Work out the finished part from the listing and answer in its coordinate system (mm). Give positions to 0.01 mm unless a question says otherwise; leave off trailing zeros. Order: outer loops, then holes, each group sorted by start corner. A loop starts at its lowest first (then second) coordinate and runs counter-clockwise, first axis right, second up. Notation, with made-up numbers: M 44,30.25 L 93,30.25 A27 ccw 93,61.25 Z; hole C -16,86 d8. An arc over 180 degrees is marked long. One line per item, written item: value.
from build123d import *

# Parameters (mm, degrees)
F1_DEPTH = 75
F2_R     = 20


with BuildPart() as f1:
    # F0 (on Front) → F1 (new body, symmetric)
    with BuildSketch(Plane.XZ):
        Polygon((-6.964528, 35.829392), (0, 0), (114, 0), (93.814774, 58.622152), (59.041445, 49.304666), (49.05917, 50.840897), align=None)
    extrude(amount=F1_DEPTH, both=True)

    # F2
    f2_edges = [f1.edges().sort_by_distance(p)[0] for p in [
        (49.05917, 0, 50.840897),
        (59.041445, 0, 49.304666),
    ]]
    fillet(f2_edges, radius=F2_R)


solid = f1.part
(1) Section B-B, the plane z = 13.5 is taken. Give the vertices of the cut face in (x, y).
Findings:
outline: M -2.62,-75 L 109.35,-75 L 109.35,75 L -2.62,75 Z
(2) Section A-A, the plane y = 56 is taken. Give the vertices of the cut face in (x, z), then the cut area to 3 significant figures.
Findings:
outline: M -6.96,35.83 L 0,0 L 114,0 L 93.81,58.62 L 63.1,50.39 A20 cw 54.89,49.94 L 53.22,50.2 A20 ccw 45,49.75 Z
area: 5,270 mm^2
(3) Find the intervals of material crossed by probe 1 along Z at (x, y) = (58.5, 4.5); probe 2 along X at (y, z) = (66, 8); probe 3 along X at (y, z) = (15.5, 26.5), in increasing order. Write a range as from..to.
Findings:
probe 1: z = 0..49.72
probe 2: x = -1.56..111.25
probe 3: x = -5.15..104.88
(4) Determine the mould class of faces 1 (the flat face through (53, 75, 23)), 2 (the flat face through (-3.53, -1.05, 18.17)), 3 (the cylindrical face through (49, 1, 50.4)) for opening direction X: pulls with the +X half, pulls with the -X half, needs draft (parallel to the pull), parting line crosses it, or undercut.
Findings:
face 1: needs draft
face 2: pulls with the -X half
face 3: undercut
(5) Section C-C, the plane x = 60.5 is taken. Give the vertices of the cut face in (y, z), then the cut area to 3 significant figures.
Findings:
outline: M -75,0 L 75,0 L 75,49.88 L -75,49.88 Z
area: 7,480 mm^2
(6) Given P1, Ø4, axis at y = -45, z = 50, coming from the +X side; P2, Ø1, axis at x = 53, y = -10.5, coming from the +Z side; P3, Ø10, axis at y = 54, z = 18.5, coming from the +X side, each flat-ended and moving along its own axis, determine where each tip first touches the part or whether it passes through.
Findings:
P1: stops at x = 97.47
P2: stops at z = 50.3
P3: stops at x = 109.35
